Check sheet for the modelled part. Datum: model origin and axes. Units: mm. A direction names the side the tool comes from. Coordinates: 2 decimals unless noted, no trailing zeros. Loops run counter-clockwise (first coordinate to the right, second up) from the corner with the lowest first, then second, coordinate; pieces in that order, holes last. Notation, with made-up numbers: (-39.75, 33.25) -> (-19.75, 33.25) arc R28 cw to (-19.75, 57.25) -> close; hole circle Ø9 at (-15.5, -2). An arc over 180 degrees is marked (long way). Use CSV: the item, a comma, the result in double quotes.
```python
from build123d import *

# Parameters (mm, degrees)
F0_W     = 13
F0_H     = 8
F1_DEPTH = 25
F2_W     = 11
F2_H     = 6
F3_DEPTH = 1
F4_W     = 2
F4_H     = 2
F5_DEPTH = 3


with BuildPart() as f1:
    # F0 (on Top) → F1 (new body)
    with BuildSketch(Plane.XY):
        Rectangle(F0_W, F0_H)
    extrude(amount=F1_DEPTH)

    # F2 (on face) → F3 (cut)
    with BuildSketch(Plane(origin=(0, 0, 0), x_dir=(1, 0, 0), z_dir=(0, 0, -1))):
        Rectangle(F2_W, F2_H)
    extrude(amount=-F3_DEPTH, mode=Mode.SUBTRACT)

    # F4 (on face) → F5 (cut)
    with BuildSketch(Plane.XZ.offset(4)):
        with Locations((0, 18)):
            Rectangle(F4_W, F4_H)
    extrude(amount=-F5_DEPTH, mode=Mode.SUBTRACT)


solid = f1.part
```
1) Cross-section at B-B on x = 2.5. Record the boundary of the cut face in (y, z).
Answer below:
outline,"(-4, 0) -> (-3, 0) -> (-3, 1) -> (3, 1) -> (3, 0) -> (4, 0) -> (4, 25) -> (-4, 25) -> close"
2) Draft check along Y on faces 1 (the flat face through (-6.5, 0, 12)), 2 (the flat face through (0, 0, 1)), 3 (the flat face through (0, -4, 12)), 4 (the flat face through (-0.1, -3, 0.5)). Enter one of: released by +Y, released by -Y, zero draft, split by the parting line, or undercut.
Answer below:
face 1,"zero draft"
face 2,"undercut"
face 3,"released by -Y"
face 4,"undercut"
3) Cross-section at D-D on x = -0.75. Record the boundary of the cut face in (y, z), and give its area (3 significant figures).
Answer below:
outline,"(-4, 0) -> (-3, 0) -> (-3, 1) -> (3, 1) -> (3, 0) -> (4, 0) -> (4, 25) -> (-4, 25) -> (-4, 19) -> (-1, 19) -> (-1, 17) -> (-4, 17) -> close"
area,"188 mm²"
4) Thickness scan on line 1 along Z through (x, y) = (2.25, -1.5); line 2 along Z through (x, y) = (0.5, -3.5); line 3 along Y through (x, z) = (-0.5, 17.75). Record the ranges inside material, lowest first. Write a range as from..to.
Answer below:
line 1,"z = 1..25"
line 2,"z = 0..17, 19..25"
line 3,"y = -1..4"
5) Access from +Z, -Z, +X, -X, +Y, -Y to the whole of each face (thin tool, end or side, straight path). Record for faces 5 (the flat face through (0, -3, 19)), 6 (the flat face through (-5.5, 0, 0.5)), 7 (the flat face through (0, 4, 12)).
Answer below:
face 5,"-Y"
face 6,"-Z"
face 7,"+Z, -Z, +X, -X, +Y"
6) Go/stop test with flat-tipped pins: pin 1 Ø0.6 at (x, y) = (0.5, -2) entering from -Z; pin 2 Ø1 at (x, z) = (0, 18) entering from -Y. Record where each tip stops, or that it passes through.
Answer below:
pin 1,"stops at z = 1"
pin 2,"stops at y = -1"
7) Cross-section at C-C on y = -2.25. Record the boundary of the cut face in (x, z).
Answer below:
outline,"(-6.5, 0) -> (-5.5, 0) -> (-5.5, 1) -> (5.5, 1) -> (5.5, 0) -> (6.5, 0) -> (6.5, 25) -> (-6.5, 25) -> close; hole (-1, 17) -> (1, 17) -> (1, 19) -> (-1, 19) -> close"
8) Cross-section at A-A on z = 18.5. Record the boundary of the cut face in (x, y), and give its area (3 significant figures).
Answer below:
outline,"(-6.5, -4) -> (-1, -4) -> (-1, -1) -> (1, -1) -> (1, -4) -> (6.5, -4) -> (6.5, 4) -> (-6.5, 4) -> close"
area,"98.0 mm²"
